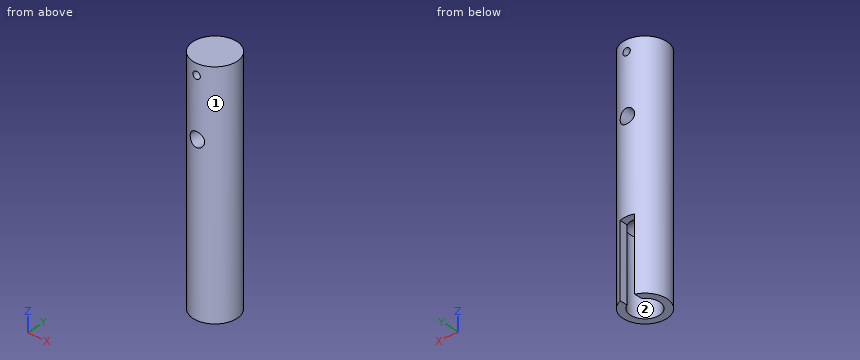
Autodesk Inventor part; units mm, degrees
ref_plane "作業平面1" through (0, 6, 0) normal (0, 1, 0) x (-1, 0, 0)
ref_plane "YZ Plane" through (0, 0, 0) normal (1, 0, 0) x (0, 1, 0)
ref_plane "XY Plane" through (0, 0, 0) normal (0, 0, 1) x (1, 0, 0)
sketch "スケッチ1" plane through (0, 0, 0) normal (0, 0, 1) x (1, 0, 0)
  circle A0 centre (0, 0) radius 6
  dimension "d0" = 12
extrude "押し出し1" add sketch "スケッチ1" along normal blind 64
ref_plane "作業平面1" through (0, 6, 0) normal (0, 1, 0) x (-1, 0, 0)
sketch "スケッチ2" plane through (0, 6, 0) normal (0, 1, 0) x (-1, 0, 0)
  line L0 (0, 0) -> (2, 0)
  line L1 (2, 0) -> (2, 20)
  line L2 (2, 20) -> (0, 20)
  line L3 (0, 20) -> (0, 0)
  line L4 (6, 0) -> (-6, 0)
  line L5 (0, 20) -> (-2, 20)
  line L6 (-2, 20) -> (-2, 0)
  line L7 (-2, 0) -> (0, 0)
  line L8 (0, 0) -> (0, 20)
  dimension "d3" = 2
  dimension "d4" = 20
  dimension "d5" = 2
  dimension "d31" = 4
extrude "押し出し2" cut sketch "スケッチ2" against normal blind 6
sketch "スケッチ3" plane through (0, 0, 0) normal (0, 0, -1) x (-1, 0, 0)
  point P0 (0, 0)
  point P1 (0, 0)
hole "穴1" at (0, 0, 0) direction (0, 0, 1) diameter 8 depth 20 tip angle 118
sketch "スケッチ4" plane through (0, 6, 0) normal (0, 1, 0) x (-1, 0, 0)
  line L0 (2, 20) -> (-2, 20)
  point P0 (0, 0)
  point P1 (0, 45)
  dimension "d15" = 25
hole "穴2" at (0, 6, 45) direction (0, -1, 0) diameter 4 end through all
sketch "スケッチ5" plane through (0, 6, 0) normal (0, 1, 0) x (-1, 0, 0)
  line L0 (6, 64) -> (-6, 64)
  point P0 (0, 0)
  point P1 (0, 61)
  dimension "d23" = 3
hole "穴3" at (0, 6, 61) direction (0, -1, 0) diameter 2 end through all
properties part number "small_bar_motor" material "アルミニウム 6061-AHC"
The listing builds one solid part. Answer for the finished solid, in the listing's coordinates (mm). Face numbers are marked on the shaded views. A direction names the side the tool comes from. Coordinates: 2 decimals unless noted, no trailing zeros. Loops run counter-clockwise (first coordinate to the right, second up) from the corner with the lowest first, then second, coordinate; pieces in that order, holes last. Notation, with made-up numbers: (49.25, 68) -> (104.25, 68) arc R20 ccw to (104.25, 90) -> close; hole circle Ø1 at (-36.75, 53.25). An arc over 180 degrees is marked (long way). Use one line per item in the form item = value. Start each with the question number.
Item 1: Flat-ended cylindrical pins translate along their axes: pin 1 Ø0.8 at (x, y) = (1, 4.5) entering from -Z; pin 2 Ø1.6 at (x, z) = (0, 61) entering from +Y; pin 3 Ø6 at (x, z) = (-3.5, 45.5) entering from -Y; pin 4 Ø2.5 at (y, z) = (5, 10.5) entering from +X. Find the tip coordinate at first contact, or state that the pin passes through.
Item 2: The part is cut by section C-C on y = 2.25. Count the separate pieces of the cut face and the enclosed holes in it, then the cut area to 3 significant figures.
Item 3: The part is cut by section A-A on z = 45. Determine the outline of the cut face in (x, y).
Item 4: The part is cut by section D-D on x = 5.25. Determine the outline of the cut face in (y, z), then the cut area to 3 significant figures.
Item 5: A tool of negligible diameter and unlimited length cuts with its end or side. For the marked faces 1 and 2, from which of +Z, -Z, +X, -X, +Y, -Y can it reach the whole face along a straight path? Write none if from no direction.
Item 6: The part is cut by section B-B on z = 5. Determine the outline of the cut face in (x, y).
Item 7: Consider L1, parallel to Z at x = 0, y = -3; L2, parallel to Z at x = 0, y = -2.5; L3, parallel to Z at x = -1.25, y = -3. Determine where each line is inside the solid, lowest interval first. Write a range as [from, to].
Answer key:
q1.pin_1 = 20
q1.pin_2 = through
q1.pin_3 = -5.95
q1.pin_4 = 4.68
q2.separate_pieces = 1
q2.enclosed_holes = 2
q2.area = 560 mm2
q3.outline = (-2, -5.66) -> (-2, 5.66) arc R6 ccw to start; (2, -5.66) arc R6 ccw to (2, 5.66) -> close
q4.outline = (-2.9, 0) -> (2.9, 0) -> (2.9, 64) -> (-2.9, 64) -> close
q4.area = 372 mm2
q5.face_1 = +Z, -Z
q5.face_2 = -Z
q6.outline = (-2, 3.46) -> (-2, 5.66) arc R6 ccw (long way) to (2, 5.66) -> (2, 3.46) arc R4 cw (long way) to start
q7.L1 = [20.6, 43], [47, 60], [62, 64]
q7.L2 = [20.9, 43], [47, 60], [62, 64]
q7.L3 = [20.45, 43.44], [46.56, 64]
